Check sheet for the modelled part. Datum: model origin and axes. Units: mm. Face numbers are marked on the shaded views. A direction names the side the tool comes from. Coordinates: 2 decimals unless noted, no trailing zeros. Loops run counter-clockwise (first coordinate to the right, second up) from the corner with the lowest first, then second, coordinate; pieces in that order, holes last. Notation, with made-up numbers: (-12, -9) -> (41, -9) arc R17 cw to (41, 20) -> close; hole circle Ø7 at (74, -21.75). An arc over 180 degrees is marked (long way). Use one line per item in the form item = value.
Autodesk Inventor part; units mm, degrees
ref_plane "mgn_screw1_XY" through (22.5, 16.5, 0) normal (0, 0, 1) x (1, 0, 0)
ref_plane "mgn_screw1_YZ" through (22.5, 16.5, 0) normal (1, 0, 0) x (0, 1, 0)
ref_plane "mgn_screw1_ZX" through (22.5, 16.5, 0) normal (0, 1, 0) x (0, 0, 1)
sketch "Sketch_1" plane through (0, 0, 0) normal (0, 0, 1) x (1, 0, 0)
  line L0 (-28.5, 0) -> (28.5, 0)
  line L1 (28.5, 0) -> (28.5, 31)
  line L2 (28.5, 31) -> (-28.5, 31)
  line L3 (-28.5, 31) -> (-28.5, 0)
extrude "Extrusion1" add sketch "Sketch_1" along normal blind 2.3
sketch "Sketch_3" plane through (0, 16.5, 0) normal (0, 1, 0) x (1, 0, 0)
  line L0 (22.5, -2.3) -> (22.5, 0)
  line L1 (22.5, 0) -> (24, 0)
  line L2 (24, 0) -> (23.7295, -0.2705)
  line L3 (23.7295, -0.2705) -> (23.7295, -2.0295)
  line L4 (23.7295, -2.0295) -> (24, -2.3)
  line L5 (24, -2.3) -> (22.5, -2.3)
  line L6 (22.5, -2.3) -> (22.5, 0)
revolve "Revolution1" cut sketch "Sketch_3" angle 360 about axis through (22.5, 16.5, 2.3) along (0, 0, 1)
thread "Thread1"
sketch "Sketch_2" plane through (0, 16.5, 0) normal (0, 1, 0) x (1, 0, 0)
  line L0 (-22.5, -2.3) -> (-22.5, 0)
  line L1 (-22.5, 0) -> (-21, 0)
  line L2 (-21, 0) -> (-21.2705, -0.2705)
  line L3 (-21.2705, -0.2705) -> (-21.2705, -2.0295)
  line L4 (-21.2705, -2.0295) -> (-21, -2.3)
  line L5 (-21, -2.3) -> (-22.5, -2.3)
  line L6 (-22.5, -2.3) -> (-22.5, 0)
revolve "Revolution2" cut sketch "Sketch_2" angle 360 about axis through (-22.5, 16.5, 2.3) along (0, 0, 1)
thread "Thread2"
sketch "Sketch_10" plane through (0, 0, 0) normal (0, 0, 1) x (1, 0, 0)
  line L0 (-28.5, 0) -> (28.5, 0)
  line L1 (28.5, 0) -> (28.5, 2.3)
  line L2 (28.5, 2.3) -> (-28.5, 2.3)
  line L3 (-28.5, 2.3) -> (-28.5, 0)
extrude "Extrusion2" add sketch "Sketch_10" along normal blind 21
sketch "Sketch_11" plane through (0, 0, 14) normal (0, 0, 1) x (1, 0, 0)
  line L0 (20, 0) -> (20, 2.3)
  line L1 (20, 2.3) -> (22.1, 2.3)
  line L2 (22.1, 2.3) -> (22.1, 0)
  line L3 (22.1, 0) -> (20, 0)
  line L4 (20, 0) -> (20, 2.3)
revolve "Revolution3" cut sketch "Sketch_11" angle 360 about axis through (20, 0, 14) along (0, -1, 0)
sketch "Sketch_12" plane through (0, 0, 14) normal (0, 0, 1) x (1, 0, 0)
  line L0 (-20, 0) -> (-20, 2.3)
  line L1 (-20, 2.3) -> (-17.9, 2.3)
  line L2 (-17.9, 2.3) -> (-17.9, 0)
  line L3 (-17.9, 0) -> (-20, 0)
  line L4 (-20, 0) -> (-20, 2.3)
revolve "Revolution4" cut sketch "Sketch_12" angle 360 about axis through (-20, 0, 14) along (0, -1, 0)
ref_plane "mgn_screw1_XY" through (22.5, 16.5, 0) normal (0, 0, 1) x (1, 0, 0)
ref_plane "mgn_screw1_YZ" through (22.5, 16.5, 0) normal (1, 0, 0) x (0, 1, 0)
ref_plane "mgn_screw1_ZX" through (22.5, 16.5, 0) normal (0, 1, 0) x (0, 0, 1)
ref_plane "mgn_screw2_XY" through (-22.5, 16.5, 0) normal (0, 0, 1) x (1, 0, 0)
ref_plane "mgn_screw2_YZ" through (-22.5, 16.5, 0) normal (1, 0, 0) x (0, 1, 0)
ref_plane "mgn_screw2_ZX" through (-22.5, 16.5, 0) normal (0, 1, 0) x (0, 0, 1)
ref_plane "plate_screw1_XY" through (-20, 0, 14) normal (0, 1, 0) x (1, 0, 0)
ref_plane "plate_screw1_YZ" through (-20, 0, 14) normal (1, 0, 0) x (0, 0, -1)
ref_plane "plate_screw1_ZX" through (-20, 0, 14) normal (0, 0, -1) x (0, 1, 0)
ref_plane "plate_screw2_XY" through (20, 0, 14) normal (0, 1, 0) x (1, 0, 0)
ref_plane "plate_screw2_YZ" through (20, 0, 14) normal (1, 0, 0) x (0, 0, -1)
ref_plane "plate_screw2_ZX" through (20, 0, 14) normal (0, 0, -1) x (0, 1, 0)
properties part number "ME5-5"
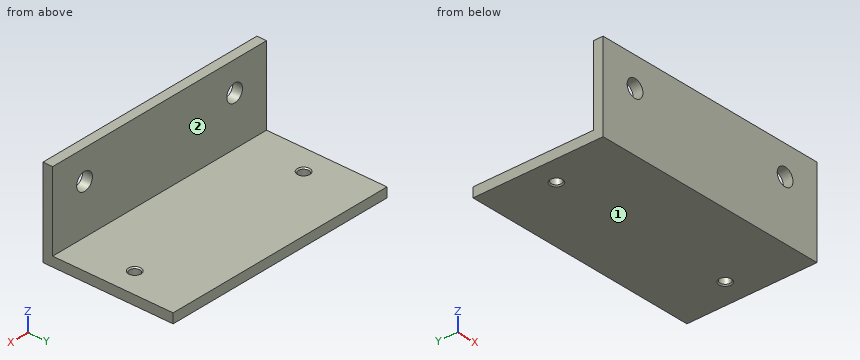
(1) Scan lines: line 1 along Y through (x, z) = (22.5, 1.15); line 2 along Y through (x, z) = (7.5, 15); line 3 along Z through (x, y) = (-20, 1.8). Record each from-to range of solid material in increasing order.
Established:
line_1 = 0 to 15.27, 17.73 to 31
line_2 = 0 to 2.3
line_3 = 0 to 11.9, 16.1 to 21
(2) Go/stop test with flat-tipped pins: P1, Ø8, axis at x = -5.5, z = 15.5, coming from the -Y side; P2, Ø1, axis at x = 6.5, y = 27.5, coming from the +Z side; P3, Ø9.5, axis at x = -1.5, z = 13.5, coming from the +Y side. Record where each tip stops, or that it passes through.
Established:
P1 = 0
P2 = 2.3
P3 = 2.3
(3) Section check B-B, the plane x = 20. Record the boundary of the cut face in (y, z), plus the area to 3 significant figures.
Established:
outline = (0, 0) -> (31, 0) -> (31, 2.3) -> (2.3, 2.3) -> (2.3, 11.9) -> (0, 11.9) -> close; (0, 16.1) -> (2.3, 16.1) -> (2.3, 21) -> (0, 21) -> close
area = 105 mm²
(4) Section check C-C, the plane z = 14. Record the boundary of the cut face in (x, y).
Established:
outline = (-28.5, 0) -> (-22.1, 0) -> (-22.1, 2.3) -> (-28.5, 2.3) -> close; (-17.9, 0) -> (17.9, 0) -> (17.9, 2.3) -> (-17.9, 2.3) -> close; (22.1, 0) -> (28.5, 0) -> (28.5, 2.3) -> (22.1, 2.3) -> close
(5) Section check D-D, the plane x = -6. Record the boundary of the cut face in (y, z).
Established:
outline = (0, 0) -> (31, 0) -> (31, 2.3) -> (2.3, 2.3) -> (2.3, 21) -> (0, 21) -> close
(6) Section check A-A, the plane y = 16.5. Record the boundary of the cut face in (x, z).
Established:
outline = (-28.5, 0) -> (-24, 0) -> (-23.73, 0.27) -> (-23.73, 2.03) -> (-24, 2.3) -> (-28.5, 2.3) -> close; (-21.27, 0.27) -> (-21, 0) -> (21, 0) -> (21.27, 0.27) -> (21.27, 2.03) -> (21, 2.3) -> (-21, 2.3) -> (-21.27, 2.03) -> close; (23.73, 0.27) -> (24, 0) -> (28.5, 0) -> (28.5, 2.3) -> (24, 2.3) -> (23.73, 2.03) -> close
(7) Tool access check on the marked faces 1 and 2. Record the directions out of +Z, -Z, +X, -X, +Y, -Y that give a thin tool (end or side, any length) a straight path to the whole face; none if there is none.
Established:
face_1 = -Z, +X, -X, +Y, -Y
face_2 = +Z, +X, -X, +Y
